```python
from build123d import *

# Parameters (mm, degrees)
SKETCH1_W                 = 107
SKETCH1_H                 = 25
SKETCH1_W_2               = 86.65
SKETCH1_H_2               = 7.4399
BOSS_EXTRUDE1_DEPTH       = 1.692
FILLET1_R                 = 1
F_2_CLEARANCE_HOLE1_D     = 2.4384
F_2_CLEARANCE_HOLE1_DEPTH = 8.66
F_2_CLEARANCE_HOLE1_TIP   = 0.732569267
SKETCH10_R                = 0.8
SKETCH10_R_2              = 0.4064
CUT_EXTRUDE1_DEPTH        = 10
SKETCH11_R                = 0.254
SKETCH11_R_2              = 0.23
CUT_EXTRUDE2_DEPTH        = 2.692


with BuildPart() as part:
    # Sketch1 → Boss-Extrude1 (new body)
    with BuildSketch(Plane.XY):
        Rectangle(SKETCH1_W, SKETCH1_H)
        with Locations((8.175, 7.78005)):
            Rectangle(SKETCH1_W_2, SKETCH1_H_2, mode=Mode.SUBTRACT)
        with Locations((8.175, -7.78005)):
            Rectangle(SKETCH1_W_2, SKETCH1_H_2, mode=Mode.SUBTRACT)
        with Locations((8.175, -7.78005)):
            Rectangle(SKETCH1_W_2, SKETCH1_H_2)
        with Locations((8.175, 7.78005)):
            Rectangle(SKETCH1_W_2, SKETCH1_H_2)
    extrude(amount=BOSS_EXTRUDE1_DEPTH)

    # Fillet1
    fillet1_edges = [part.edges().sort_by_distance(p)[0] for p in [
        (53.5, -12.5, 0.846),
        (-53.5, -12.5, 0.846),
        (-53.5, 12.5, 0.846),
        (53.5, 12.5, 0.846),
    ]]
    fillet(fillet1_edges, radius=FILLET1_R)

    # 2 Clearance Hole1
    with Locations(Plane(origin=(0, 0, 0), x_dir=(-1, 0, 0), z_dir=(0, 0, -1))):
        with Locations((-50, 0), (32, 0)):
            Hole(F_2_CLEARANCE_HOLE1_D / 2, depth=F_2_CLEARANCE_HOLE1_DEPTH)
            with Locations((0, 0, -(F_2_CLEARANCE_HOLE1_DEPTH + F_2_CLEARANCE_HOLE1_TIP / 2))):  # 118° drill point
                Cone(0, F_2_CLEARANCE_HOLE1_D / 2, F_2_CLEARANCE_HOLE1_TIP, mode=Mode.SUBTRACT)

    # Sketch10 → Cut-Extrude1 (cut)
    with BuildSketch(Plane(origin=(0, 0, 0), x_dir=(-1, 0, 0), z_dir=(0, 0, -1))):
        with Locations((37.675, -6.925)):
            Circle(SKETCH10_R)
        with Locations((37.675, 1.575)):
            Circle(SKETCH10_R)
        with Locations((37.05, 10.35)):
            Circle(SKETCH10_R_2)
        with Locations((38.875, 10.35)):
            Circle(SKETCH10_R_2)
        with Locations((40.975, 10.35)):
            Circle(SKETCH10_R_2)
        with BuildLine():
            Line((48.244, -4.806), (47.506, -4.806))
            ThreePointArc((47.506, -4.806), (47.125, -4.425), (47.506, -4.044))
            Line((47.506, -4.044), (48.244, -4.044))
            ThreePointArc((48.244, -4.044), (48.625, -4.425), (48.244, -4.806))
        make_face()
        with BuildLine():
            Line((48.244, -9.806), (47.506, -9.806))
            ThreePointArc((47.506, -9.806), (47.125, -9.425), (47.506, -9.044))
            Line((47.506, -9.044), (48.244, -9.044))
            ThreePointArc((48.244, -9.044), (48.625, -9.425), (48.244, -9.806))
        make_face()
        with BuildLine():
            Line((47.506, -0.544), (48.244, -0.544))
            ThreePointArc((48.244, -0.544), (48.625, -0.925), (48.244, -1.306))
            Line((48.244, -1.306), (47.506, -1.306))
            ThreePointArc((47.506, -1.306), (47.125, -0.925), (47.506, -0.544))
        make_face()
        with BuildLine():
            Line((47.506, 4.456), (48.244, 4.456))
            ThreePointArc((48.244, 4.456), (48.625, 4.075), (48.244, 3.694))
            Line((48.244, 3.694), (47.506, 3.694))
            ThreePointArc((47.506, 3.694), (47.125, 4.075), (47.506, 4.456))
        make_face()
    extrude(amount=-CUT_EXTRUDE1_DEPTH, mode=Mode.SUBTRACT)

    # Sketch11 → Cut-Extrude2 (cut, through all)
    with BuildSketch(Plane(origin=(0, 0, 0), x_dir=(-1, 0, 0), z_dir=(0, 0, -1))):
        with Locations((27.85, -9.05005)):
            Circle(SKETCH11_R)
        with Locations((22.77, -6.51005)):
            Circle(SKETCH11_R)
        with Locations((17.69, -9.05005)):
            Circle(SKETCH11_R)
        with Locations((12.61, -6.51005)):
            Circle(SKETCH11_R)
        with Locations((17.69, 6.51005)):
            Circle(SKETCH11_R_2)
        with Locations((12.61, 9.05005)):
            Circle(SKETCH11_R_2)
        with Locations((7.53, -9.05005)):
            Circle(SKETCH11_R)
        with Locations((2.45, -6.51005)):
            Circle(SKETCH11_R)
        with Locations((7.53, 6.51005)):
            Circle(SKETCH11_R_2)
        with Locations((2.45, 9.05005)):
            Circle(SKETCH11_R_2)
        with Locations((-2.63, -9.05005)):
            Circle(SKETCH11_R)
        with Locations((-7.71, -6.51005)):
            Circle(SKETCH11_R)
        with Locations((-2.63, 6.51005)):
            Circle(SKETCH11_R_2)
        with Locations((-7.71, 9.05005)):
            Circle(SKETCH11_R_2)
        with Locations((-12.79, -9.05005)):
            Circle(SKETCH11_R)
        with Locations((-17.87, -6.51005)):
            Circle(SKETCH11_R)
        with Locations((27.85, 6.51005)):
            Circle(SKETCH11_R_2)
        with Locations((22.77, 9.05005)):
            Circle(SKETCH11_R_2)
        with Locations((-12.79, 6.51005)):
            Circle(SKETCH11_R_2)
        with Locations((-17.87, 9.05005)):
            Circle(SKETCH11_R_2)
        with Locations((-22.95, -9.05005)):
            Circle(SKETCH11_R)
        with Locations((-28.03, -6.51005)):
            Circle(SKETCH11_R)
        with Locations((-22.95, 6.51005)):
            Circle(SKETCH11_R_2)
        with Locations((-28.03, 9.05005)):
            Circle(SKETCH11_R_2)
        with Locations((-33.11, -9.05005)):
            Circle(SKETCH11_R)
        with Locations((-38.19, -6.51005)):
            Circle(SKETCH11_R)
        with Locations((-33.11, 6.51005)):
            Circle(SKETCH11_R_2)
        with Locations((-38.19, 9.05005)):
            Circle(SKETCH11_R_2)
        with Locations((-43.27, -9.05005)):
            Circle(SKETCH11_R)
        with Locations((-48.35, -6.51005)):
            Circle(SKETCH11_R)
        with Locations((-43.27, 6.51005)):
            Circle(SKETCH11_R_2)
        with Locations((-48.35, 9.05005)):
            Circle(SKETCH11_R_2)
    extrude(amount=-CUT_EXTRUDE2_DEPTH, mode=Mode.SUBTRACT)


solid = part.part
```
Design review of the part built by this model. Coordinates are the model's own, in mm. Coordinates: 2 decimals unless noted, no trailing zeros. Order: outer loops, then holes, each group sorted by start corner. A loop starts at its lowest first (then second) coordinate and runs counter-clockwise, first axis right, second up.
1) Wall thickness on line 1 along Y through (x, z) = (7.71, 0.5); line 2 along X through (y, z) = (-4.5, 1.35); line 3 along X through (y, z) = (-0.5, 1.1): over which ranges is each line inside the solid? List them lowest first.
2) Mouldability with a two-part tool opening along X and no side actions: class faces 1 (the flat face through (53.5, 0, 1)), 2 (the flat face through (-1, 12.5, 1)), 3 (the cylindrical face through (-30.84, 0.37, 0.86)) as +X half, -X half, draft (parallel to the pull), parting line (faces both ways), or undercut.
3) Clearance check with a flat-ended pin moving along its axis: pin 1 (2 mm diameter, centred on x = 50, y = 0, fed in from -Z). State where the tip first meets the part, or that it passes through.
4) Take a section at A-A, the plane x = 50. Give the boundary of the cut face in (y, z).
Returned:
1. line 1: y = -12.5 to -6.76, -6.26 to 8.82, 9.28 to 12.5
1. line 2: x = -53.5 to -48.62, -47.13 to 53.5
1. line 3: x = -53.5 to -33.11, -30.89 to 48.89, 51.11 to 53.5
2. face 1: +X half
2. face 2: draft
2. face 3: undercut
3. pin 1: passes through
4. outline: (-12.5, 0) - (-1.22, 0) - (-1.22, 1.69) - (-12.5, 1.69) - close; (1.22, 0) - (12.5, 0) - (12.5, 1.69) - (1.22, 1.69) - close
